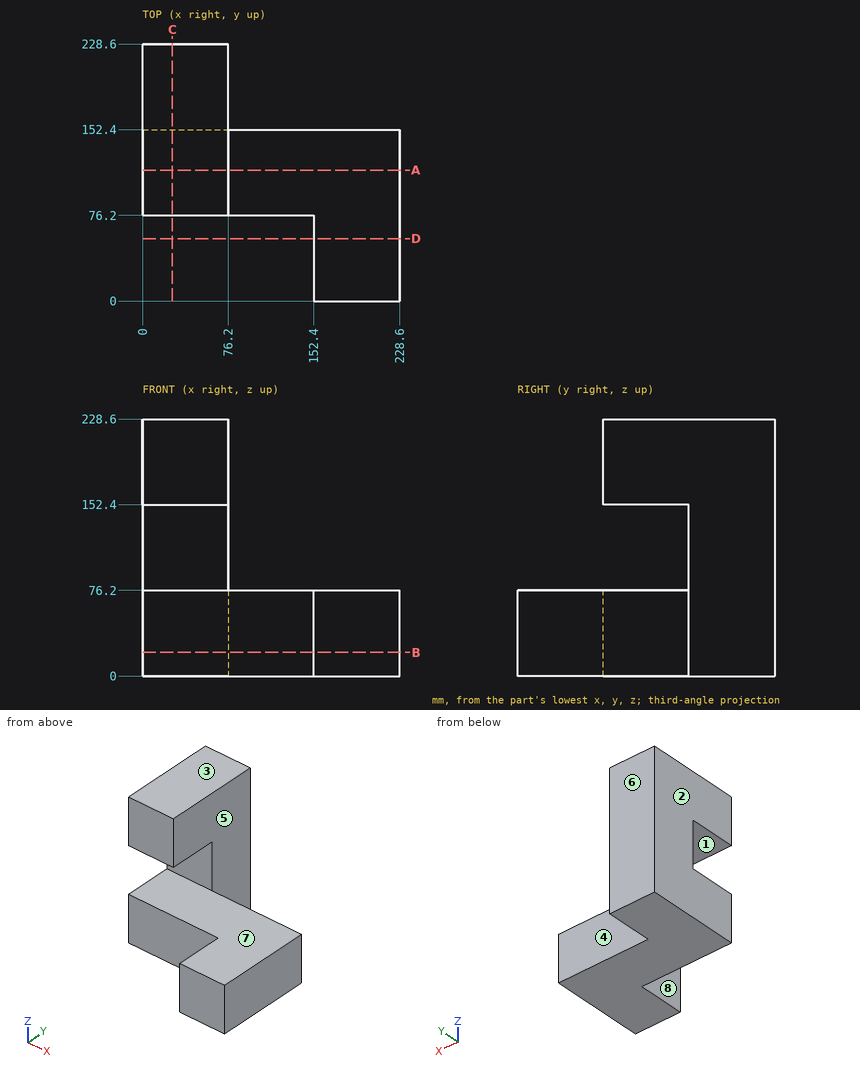
Geometry check sheet. Reference: drawing and pictorial views, mm from the part's lowest x, y, z. A direction names the side the tool comes from. Give positions to 0.01 mm unless a question says otherwise; leave off trailing zeros. Write each loop counter-clockwise with the first axis right and the second up, starting at its lowest first coordinate (ties: lowest second). Pieces come first, ordered by that corner, then holes.
Item 1: Access from +Z, -Z, +X, -X, +Y, -Y to the whole of each face (thin tool, end or side, straight path). Record for the marked faces 4, 5, 6, 7 and 8.
Item 2: Cross-section at D-D (y = 55.5). Enter the section's corners in (x, z), and give its area (3 significant figures).
Item 3: Draft check along Z on the marked faces 1, 2 and 3. Enter one of: released by +Z, released by -Z, zero draft, split by the parting line, or undercut.
Item 4: Cross-section at A-A (y = 116.5). Enter the section's corners in (x, z).
Item 5: Cross-section at B-B (z = 21). Enter the section's corners in (x, y), and give its area (3 significant figures).
Item 6: Scan lines: L1, parallel to Z at x = 41.5, y = 131; L2, parallel to Z at x = 112.5, y = 144; L3, parallel to Y at x = 165.5, z = 53.5. Record each from-to range of solid material in increasing order.
Item 7: Cross-section at C-C (x = 26.5). Enter the section's corners in (y, z).
Item 8: Gauge pin test, flat ends, axial feed: pin 1 (3 mm diameter, centred on x = 104.5, z = 25.5, fed in from -Y); pin 2 (23 mm diameter, centred on y = 55.5, z = 21.5, fed in from -X); pin 3 (23 mm diameter, centred on x = 173.5, z = 53, fed in from +Y). Record the tip position at first contact, or that the pin passes through.
Report:
1. face 4: +Z, -Z, +X, +Y
1. face 5: +Z, +X, +Y
1. face 6: +Z, -Z, +X, -X, +Y
1. face 7: +X, -X, -Y
1. face 8: +Z, -Z, -X, -Y
2. outline: (152.4, 0) - (228.6, 0) - (228.6, 76.2) - (152.4, 76.2) - close
2. area: 5,810 mm2
3. face 1: undercut
3. face 2: zero draft
3. face 3: released by +Z
4. outline: (0, 0) - (228.6, 0) - (228.6, 76.2) - (0, 76.2) - close; (0, 152.4) - (76.2, 152.4) - (76.2, 228.6) - (0, 228.6) - close
5. outline: (0, 76.2) - (152.4, 76.2) - (152.4, 0) - (228.6, 0) - (228.6, 152.4) - (76.2, 152.4) - (76.2, 228.6) - (0, 228.6) - close
5. area: 29,000 mm2
6. L1: z = 0 to 76.2, 152.4 to 228.6
6. L2: z = 0 to 76.2
6. L3: y = 0 to 152.4
7. outline: (76.2, 0) - (228.6, 0) - (228.6, 228.6) - (76.2, 228.6) - (76.2, 152.4) - (152.4, 152.4) - (152.4, 76.2) - (76.2, 76.2) - close
8. pin 1: stops at y = 76.2
8. pin 2: stops at x = 152.4
8. pin 3: stops at y = 152.4
